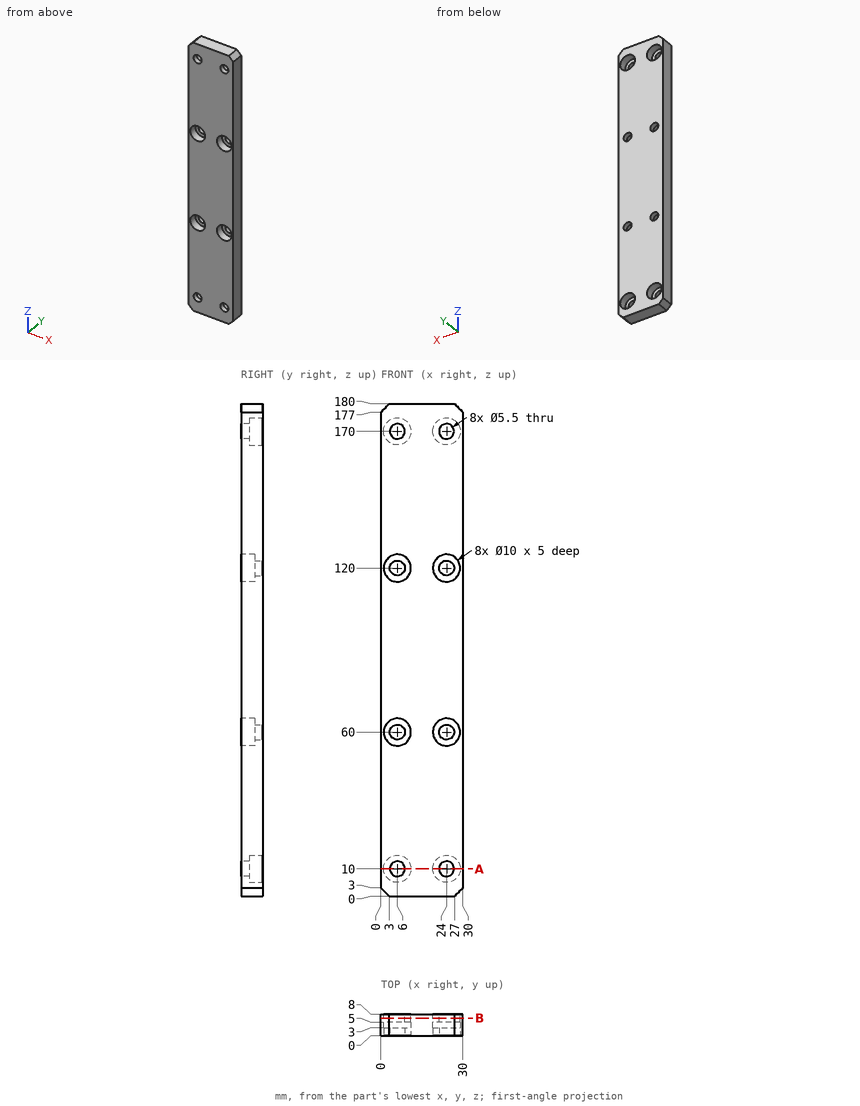
Can you work these out from the drawing? Everything is in mm from the part's minimum corner. Round coordinates to 2 decimals unless told otherwise and drop trailing zeros. Loops run counter-clockwise (first coordinate to the right, second up) from the corner with the lowest first, then second, coordinate; pieces in that order, holes last. Notation, with made-up numbers: (27, -18) - (49, -18) arc R33 ccw to (49, 20) - close; hole circle Ø5 at (15, 70.25). An arc over 180 degrees is marked (long way). Write item = value, one per line. Start each with the question number.
(1) For P1, Ø6.5, axis at x = 24, z = 60, coming from the -Y side; P2, Ø5, axis at x = 6, z = 60, coming from the -Y side; P3, Ø3, axis at x = 26, z = 10.5, coming from the +Y side, each with a flat end and sliding along its axis, tell me the tip position at first contact or that it passes through.
(2) If we section it at B-B (y = 6.5): Give the number of separate pieces and of enclosed holes in the cut face, and give its area (3 significant figures).
(3) If I drill on probe 1 along Z at (x, y) = (6, 7); probe 2 along Z at (x, y) = (6, 2); probe 3 along X at (y, z) = (2.5, 58), over which ranges is the centre line in solid material (lowest first)? Write a range as [from, to].
(4) If we section it at A-A (z = 10): Please give me the cut outline in (x, y), and give its area (3 significant figures).
Ans:
q1.P1 = 5
q1.P2 = through
q1.P3 = 3
q2.separate_pieces = 1
q2.enclosed_holes = 8
q2.area = 4,970 mm²
q3.probe_1 = [0, 5], [15, 57.25], [62.75, 117.25], [122.75, 165], [175, 180]
q3.probe_2 = [0, 7.25], [12.75, 55], [65, 115], [125, 167.25], [172.75, 180]
q3.probe_3 = [0, 1.42], [10.58, 19.42], [28.58, 30]
q4.outline = (0, 0) - (3.25, 0) - (3.25, 3) - (1, 3) - (1, 8) - (0, 8) - close; (8.75, 0) - (21.25, 0) - (21.25, 3) - (19, 3) - (19, 8) - (11, 8) - (11, 3) - (8.75, 3) - close; (26.75, 0) - (30, 0) - (30, 8) - (29, 8) - (29, 3) - (26.75, 3) - close
q4.area = 107 mm²
